Geometry check sheet. Reference: drawing and pictorial views, mm from the part's lowest x, y, z. Round coordinates to 2 decimals unless told otherwise and drop trailing zeros. Order: outer loops, then holes, each group sorted by start corner. A loop starts at its lowest first (then second) coordinate and runs counter-clockwise, first axis right, second up. Notation, with made-up numbers: M 87.25,4.25 L 124.25,4.25 A4 cw 124.25,10.25 Z; hole C 85,7.25 d6. An arc over 180 degrees is marked long. Answer as a JSON object with one key per item and string values. Group by question number.
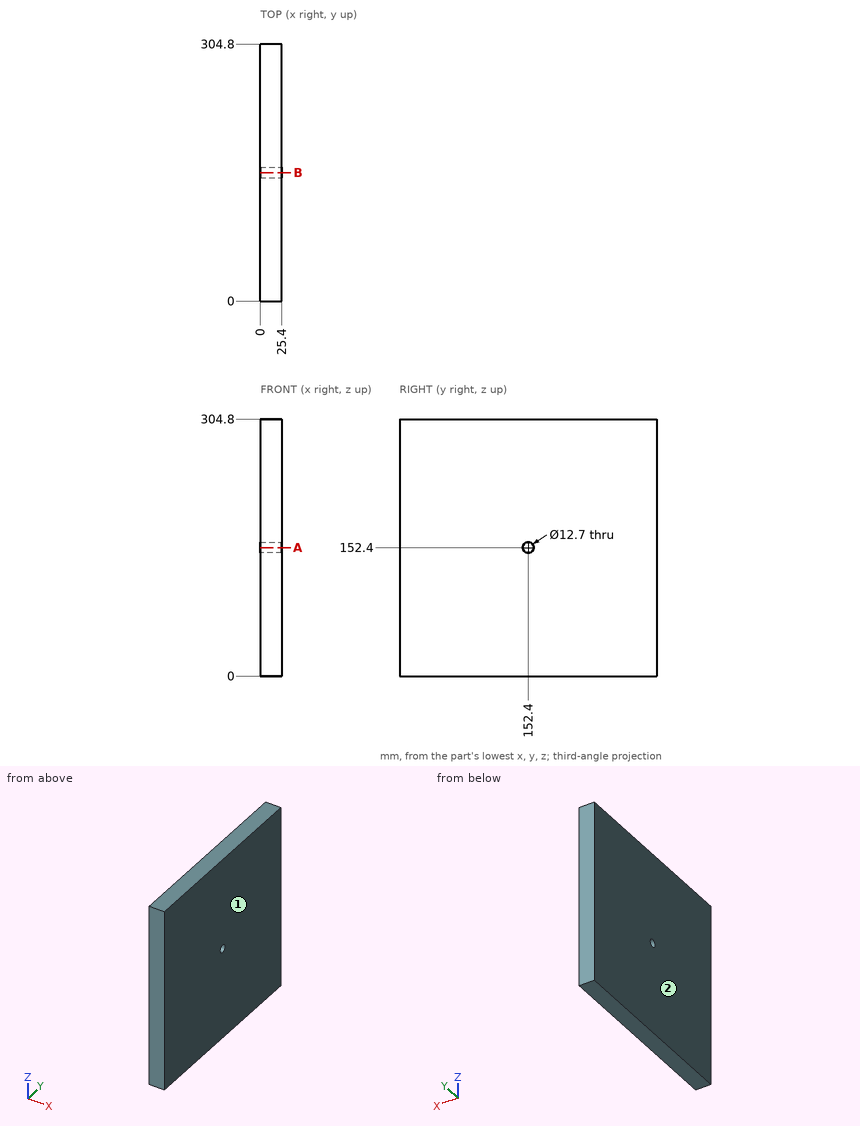
Q1. Thickness scan on line 1 (Y direction, x = 7.75, z = 152.4). Record the ranges inside material, lowest first. Write a range as from..to.
Q2. Release check for a two-part mould opening along X. For the marked faces 1 and 2 record: released by +X, released by -X, zero draft, split by the parting line, or undercut.
Q3. Cross-section at A-A, the plane z = 152.4. Record the cut outline in (x, y).
Conclusion:
{
 "1": {"line 1": "0..146.05, 158.75..304.8"},
 "2": {"face 1": "released by +X", "face 2": "released by -X"},
 "3": {"outline": "M 0,0 L 25.4,0 L 25.4,146.05 L 0,146.05 Z; M 0,158.75 L 25.4,158.75 L 25.4,304.8 L 0,304.8 Z"}
}
